Geometry: final body of the model. Coordinates: model frame, mm. A direction names the side the tool comes from. Coordinates: 2 decimals unless noted, no trailing zeros. Order: outer loops, then holes, each group sorted by start corner. A loop starts at its lowest first (then second) coordinate and runs counter-clockwise, first axis right, second up. Notation, with made-up numbers: M 71,52 L 82,52 A22 cw 82,85 Z; hole C 20,83 d1. An arc over 180 degrees is marked long. Use CSV: the item, a comma, the result in double quotes. Start each with the question number.
Q1. Section query B-B, the plane x = 6.25. Output: boundary loops of the cut face in (y, z), and give its area (3 significant figures).
Q2. Mould query, pull axis Z, two halves, no side actions, for faces 1 (the face through (28.15, 0.81, -10.68)), 2 (the face through (0.6, 0.81, -20.63)), 3 (the face through (51.07, 26, -0.81)). Classes: +Z half, -Z half, draft (parallel to the pull), parting line (faces both ways), or undercut.
Q3. Access query for faces 4 (the face through (47.5, 1, -1)), 5 (the face through (50.5, 10, -28)), 6 (the face through (59.43, 26, -0.81)), 7 (the face through (4.68, 0.57, -0.6)). Directions: +Z, -Z, +X, -X, +Y, -Y. A direction counts if a zero-diameter tool reaches every point of the face in a straight line with its end or side. Return the directions, or none.
Q4. Section query D-D, the plane y = 8.5. Output: boundary loops of the cut face in (x, z).
Q5. Section query A-A, the plane x = 30. Output: boundary loops of the cut face in (y, z).
Q6. First-contact query: P1, Ø6, axis at x = 41, z = -15, coming from the +Y side; P2, Ø1.8, axis at x = 49.5, y = 1, coming from the +Z side; P3, Ø1.8, axis at x = 7.5, y = 0.5, coming from the -Z side. Flat tips, straight axial feed; report the tip coordinate or a pass-through.
Q7. Section query C-C, the plane y = 21.6. Output: boundary loops of the cut face in (x, z).
Q8. Ray query, probe 1 along Z at (x, y) = (38, 1.35); probe 2 along Z at (x, y) = (22, 0.65); probe 3 along X at (y, z) = (13, -1.5). Return the intervals inside material, ascending.
from build123d import *

# Parameters (mm, degrees)
EXTRUDE1_DEPTH           = 1.6
SKETCH2_W                = 9.5
SKETCH2_H                = 1.6
SKETCH2_W_2              = 41
EXTRUDE2_DEPTH           = 25
SKETCH3_R                = 1.85
CUT_EXTRUDE1_DEPTH       = 72.928615584
SKETCH4_R                = 1.6
CUT_EXTRUDE2_DEPTH       = 25
CUT_EXTRUDE3_START       = -1.6
CUT_EXTRUDE3_OUTLINE_R   = 1.85
CUT_EXTRUDE3_OUTLINE_R_2 = 4
CUT_EXTRUDE3_DEPTH       = 1.6
FILLET1_R                = 2
FILLET2_R                = 2
FILLET3_R                = 2
FILLET4_R                = 2
FILLET5_R                = 2
FILLET6_R                = 2
FILLET7_R                = 2
FILLET8_R                = 2
FILLET9_R                = 2
FILLET10_R               = 2
FILLET11_R               = 2
FILLET12_R               = 2
FILLET13_R               = 2


# Read off the part's stored shape, not the designer's step: Cut-Extrude3
with BuildPart() as part:
    # Sketch1 → Extrude1 (new body)
    with BuildSketch(Plane(origin=(0, 0, 0), x_dir=(1, 0, 0), z_dir=(0, 1, 0))):
        Polygon((0, 0), (0, 21.2), (9.5, 21.2), (9.5, 29.43069384), (50.5, 29.43069384), (50.5, 21.2), (60, 21.2), (60, 0), (50.5, 0), (50.5, 4.011974119), (47.5, 4.011974119), (47.5, -3.238875216), (12.5, -3.238875216), (12.5, 4.011974119), (9.5, 4.011974119), (9.5, 0), align=None)
    extrude(amount=EXTRUDE1_DEPTH)

    # Sketch2 → Extrude2 (add)
    with BuildSketch(Plane(origin=(0, 1.6, 0), x_dir=(1, 0, 0), z_dir=(0, 1, 0))):
        with Locations((4.75, 0.8)):
            Rectangle(SKETCH2_W, SKETCH2_H)
        with Locations((55.25, 0.8)):
            Rectangle(SKETCH2_W, SKETCH2_H)
        with Locations((30, 28.63069384)):
            Rectangle(SKETCH2_W_2, SKETCH2_H)
    extrude(amount=EXTRUDE2_DEPTH)

    # Sketch3 → Cut-Extrude1 (cut, through all)
    with BuildSketch(Plane.XY):
        with Locations((6.25, 21.6)):
            Circle(SKETCH3_R)
        with Locations((6.25, 11.6)):
            Circle(SKETCH3_R)
        with Locations((53.75, 21.6)):
            Circle(SKETCH3_R)
        with Locations((53.75, 11.6)):
            Circle(SKETCH3_R)
    extrude(amount=-CUT_EXTRUDE1_DEPTH, mode=Mode.SUBTRACT)

    # Sketch4 → Cut-Extrude2 (cut)
    with BuildSketch(Plane.XY.offset(-27.83069384)):
        with Locations((20, 17.094459231)):
            Circle(SKETCH4_R)
        with Locations((40, 17.094459231)):
            Circle(SKETCH4_R)
    extrude(amount=-CUT_EXTRUDE2_DEPTH, mode=Mode.SUBTRACT)

    # Cut-Extrude3 outline → Cut-Extrude3 (cut)
    with BuildSketch(Plane.XZ.offset(CUT_EXTRUDE3_START)):
        with Locations((14, -10.761124784)):
            Circle(CUT_EXTRUDE3_OUTLINE_R)
        with Locations((22, -10.761124784)):
            Circle(CUT_EXTRUDE3_OUTLINE_R_2)
        with Locations((30, -10.761124784)):
            Circle(CUT_EXTRUDE3_OUTLINE_R)
        with Locations((22, -18.761124784)):
            Circle(CUT_EXTRUDE3_OUTLINE_R)
        with Locations((22, -2.761124784)):
            Circle(CUT_EXTRUDE3_OUTLINE_R)
        with Locations((38, -10.761124784)):
            Circle(CUT_EXTRUDE3_OUTLINE_R_2)
        with Locations((46, -10.761124784)):
            Circle(CUT_EXTRUDE3_OUTLINE_R)
        with Locations((38, -18.761124784)):
            Circle(CUT_EXTRUDE3_OUTLINE_R)
        with Locations((38, -2.761124784)):
            Circle(CUT_EXTRUDE3_OUTLINE_R)
    extrude(amount=CUT_EXTRUDE3_DEPTH, mode=Mode.SUBTRACT)

    # Fillet1
    fillet1_edges = [part.edges().sort_by_distance(p)[0] for p in [
        (47.5, 0.8, 3.238875216),
    ]]
    fillet(fillet1_edges, radius=FILLET1_R)

    # Fillet2
    fillet2_edges = [part.edges().sort_by_distance(p)[0] for p in [
        (12.5, 0.8, 3.238875216),
    ]]
    fillet(fillet2_edges, radius=FILLET2_R)

    # Fillet3
    fillet3_edges = [part.edges().sort_by_distance(p)[0] for p in [
        (60, 26.6, -0.8),
    ]]
    fillet(fillet3_edges, radius=FILLET3_R)

    # Fillet4
    fillet4_edges = [part.edges().sort_by_distance(p)[0] for p in [
        (9.5, 26.6, -0.8),
    ]]
    fillet(fillet4_edges, radius=FILLET4_R)

    # Fillet5
    fillet5_edges = [part.edges().sort_by_distance(p)[0] for p in [
        (50.5, 26.6, -28.63069384),
    ]]
    fillet(fillet5_edges, radius=FILLET5_R)

    # Fillet6
    fillet6_edges = [part.edges().sort_by_distance(p)[0] for p in [
        (50.5, 26.6, -0.8),
    ]]
    fillet(fillet6_edges, radius=FILLET6_R)

    # Fillet7
    fillet7_edges = [part.edges().sort_by_distance(p)[0] for p in [
        (0, 26.6, -0.8),
    ]]
    fillet(fillet7_edges, radius=FILLET7_R)

    # Fillet8
    fillet8_edges = [part.edges().sort_by_distance(p)[0] for p in [
        (9.5, 26.6, -28.63069384),
    ]]
    fillet(fillet8_edges, radius=FILLET8_R)

    # Fillet9
    fillet9_edges = [part.edges().sort_by_distance(p)[0] for p in [
        (0, 0.8, -21.2),
    ]]
    fillet(fillet9_edges, radius=FILLET9_R)

    # Fillet10
    fillet10_edges = [part.edges().sort_by_distance(p)[0] for p in [
        (60, 0.8, -21.2),
    ]]
    fillet(fillet10_edges, radius=FILLET10_R)

    # Fillet11
    fillet11_edges = [part.edges().sort_by_distance(p)[0] for p in [
        (30, 0, -29.43069384),
    ]]
    fillet(fillet11_edges, radius=FILLET11_R)

    # Fillet12
    fillet12_edges = [part.edges().sort_by_distance(p)[0] for p in [
        (55.25, 0, 0),
    ]]
    fillet(fillet12_edges, radius=FILLET12_R)

    # Fillet13
    fillet13_edges = [part.edges().sort_by_distance(p)[0] for p in [
        (4.75, 0, 0),
    ]]
    fillet(fillet13_edges, radius=FILLET13_R)


solid = part.part
Responses:
1,outline,"M 0,-21.2 L 1.6,-21.2 L 1.6,-1.6 L 9.75,-1.6 L 9.75,0 L 2,0 A2 ccw 0,-2 Z; M 13.45,-1.6 L 19.75,-1.6 L 19.75,0 L 13.45,0 Z; M 23.45,-1.6 L 26.6,-1.6 L 26.6,0 L 23.45,0 Z"
1,area,"61.2 mm²"
2,face 1,"undercut"
2,face 2,"-Z half"
2,face 3,"draft"
3,face 4,"+Z, +Y, -Y"
3,face 5,"-Z, +X, +Y, -Y"
3,face 6,"+Z, -Z, +X, +Y"
3,face 7,"+Z, -X, -Y"
4,outline,"M 0,-1.6 L 9.5,-1.6 L 9.5,0 L 0,0 Z; M 9.5,-29.43 L 50.5,-29.43 L 50.5,-27.83 L 9.5,-27.83 Z; M 50.5,-1.6 L 60,-1.6 L 60,0 L 50.5,0 Z"
5,outline,"M 0,-27.43 A2 ccw 2,-29.43 L 26.6,-29.43 L 26.6,-27.83 L 1.6,-27.83 L 1.6,-12.61 L 0,-12.61 Z; M 0,-8.91 L 1.6,-8.91 L 1.6,3.24 L 0,3.24 Z"
6,P1,"stops at y = 1.6"
6,P2,"stops at z = -4.01"
6,P3,"stops at z = -21.2"
7,outline,"M 0,-1.6 L 4.4,-1.6 L 4.4,0 L 0,0 Z; M 8.1,-1.6 L 9.5,-1.6 L 9.5,0 L 8.1,0 Z; M 9.5,-29.43 L 50.5,-29.43 L 50.5,-27.83 L 9.5,-27.83 Z; M 50.5,-1.6 L 51.9,-1.6 L 51.9,0 L 50.5,0 Z; M 55.6,-1.6 L 60,-1.6 L 60,0 L 55.6,0 Z"
8,probe 1,"z = -29.32 to -20.61, -16.91 to -14.76, -6.76 to -4.61, -0.91 to 3.24"
8,probe 2,"z = -28.91 to -20.61, -16.91 to -14.76, -6.76 to -4.61, -0.91 to 3.24"
8,probe 3,"x = 0 to 5.04, 7.46 to 9.5, 50.5 to 52.54, 54.96 to 60"
